Verification items for this drawing (mm, ordinates from the low corner). Round coordinates to 2 decimals unless told otherwise and drop trailing zeros. Order: outer loops, then holes, each group sorted by start corner. A loop starts at its lowest first (then second) coordinate and runs counter-clockwise, first axis right, second up. Notation, with made-up numbers: M 53.5,59 L 75.5,59 A21 ccw 75.5,82 Z; hole C 46,36 d7. An arc over 180 degrees is marked long. One line per item, written item: value. Start each with the question number.
(1) Release check for a two-part mould opening along X. For the marked faces 1, 2, 3 and 4 record: released by +X, released by -X, zero draft, split by the parting line, or undercut.
(2) Thickness scan on L1, parallel to X at y = 19, z = 29.5 (1 decimal); L2, parallel to X at y = 24.5, z = 3; L3, parallel to X at y = 27, z = 26 (1 decimal). Record the ranges inside material, lowest first.
(3) Depth check by flat-ended pin: pin 1 Ø12 at (x, y) = (64, 18.5) entering from -Z; pin 2 Ø1.5 at (x, z) = (47, 24) entering from +Y (1 decimal); pin 3 Ø2 at (x, z) = (51.5, 7) entering from -Y; pin 4 Ø1 at (y, z) = (5, 26.5) entering from -X. Enter the tip coordinate at first touch or a pass-through.
(4) Cross-section at A-A, the plane z = 32.5. Enter the section's corners in (x, y) (1 decimal).
(5) Cross-section at B-B, the plane y = 23. Enter the section's corners in (x, z) (1 decimal).
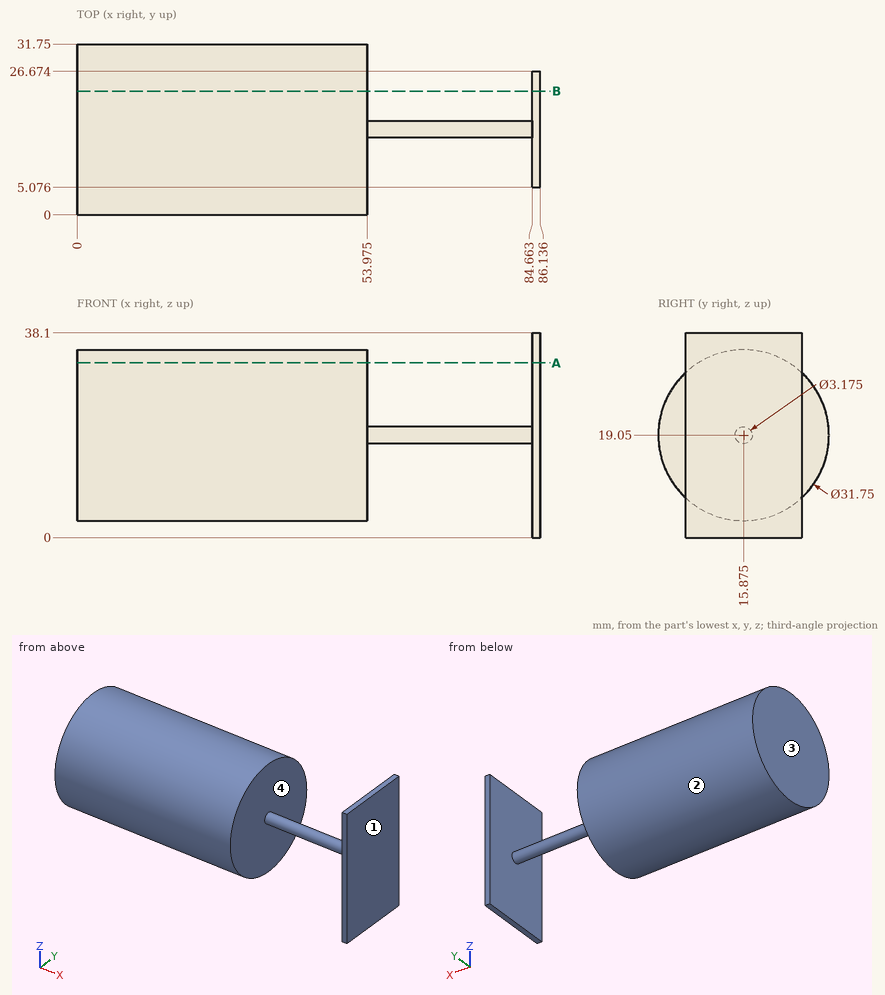
Values found:
1. face 1: released by +X
1. face 2: zero draft
1. face 3: released by -X
1. face 4: undercut
2. L1: 0 to 54, 84.7 to 86.1
2. L2: 84.66 to 86.14
2. L3: 0 to 54
3. pin 1: z = 17.46
3. pin 2: y = 31.2
3. pin 3: y = 4.48
3. pin 4: x = 0
4. outline: M 0,7.4 L 54,7.4 L 54,24.3 L 0,24.3 Z; M 84.7,5.1 L 86.1,5.1 L 86.1,26.7 L 84.7,26.7 Z
5. outline: M 0,4.9 L 54,4.9 L 54,33.2 L 0,33.2 Z; M 84.7,0 L 86.1,0 L 86.1,38.1 L 84.7,38.1 Z
